```python
from build123d import *

# Parameters (mm, degrees)
SKETCH1_R                = 10
BOSS_EXTRUDE1_DEPTH      = 8
BOSS_EXTRUDE2_DEPTH      = 1.5
FILLET1_R                = 1.6
SKETCH5_R                = 10
SKETCH5_R_2              = 8
CUT_EXTRUDE1_DEPTH       = 5
CUT_EXTRUDE2_REACH       = 19.037
SKETCH6_R                = 1.2500000000000002
CIRPATTERN1_COUNT        = 4
CUT_EXTRUDE3_DEPTH       = 17.24807680927192
FILLET2_R                = 1.6
CIRPATTERN2_COUNT        = 2
FILLET2_OF_CIRPATTERN2_R = 1.6


with BuildPart() as part:
    # Sketch1 → Boss-Extrude1 (new body)
    with BuildSketch(Plane(origin=(0, 0, 0), x_dir=(1, 0, 0), z_dir=(0, 1, 0))):
        with Locations(Location((0, 0, 0), (0, 0, 270))):
            Circle(SKETCH1_R)
    extrude(amount=BOSS_EXTRUDE1_DEPTH)

    # Sketch4 → Boss-Extrude2 (add)
    with BuildSketch(Plane(origin=(0, 8, 0), x_dir=(1, 0, 0), z_dir=(0, 1, 0))):
        with BuildLine():
            Line((-1.449999999999999, 6.336205489092031), (-1.45, 1.9124591498905275))
            ThreePointArc((-1.45, 1.9124591498905275), (-2.4, 2.9e-16), (-1.45, -1.9124591498905275))
            Line((-1.45, -1.9124591498905275), (-1.449999999999999, -6.336205489092031))
            ThreePointArc((-1.449999999999999, -6.336205489092031), (4e-16, -6.499999999999999), (1.449999999999999, -6.336205489092031))
            Line((1.449999999999999, -6.336205489092031), (1.45, -1.9124591498905275))
            ThreePointArc((1.45, -1.9124591498905275), (2.4, 0), (1.45, 1.9124591498905275))
            Line((1.45, 1.9124591498905275), (1.449999999999999, 6.336205489092031))
            ThreePointArc((1.449999999999999, 6.336205489092031), (4e-16, 6.499999999999999), (-1.449999999999999, 6.336205489092031))
        make_face()
    extrude(amount=BOSS_EXTRUDE2_DEPTH)

    # Fillet1
    fillet1_edges = [part.edges().sort_by_distance(p)[0] for p in [
        (-1.4500000000000002, 8.75, -1.9124591498905277),
        (-1.4500000000000002, 8.75, 1.9124591498905277),
        (1.4500000000000002, 8.75, 1.9124591498905277),
        (1.4500000000000002, 8.75, -1.9124591498905277),
    ]]
    fillet(fillet1_edges, radius=FILLET1_R)

    # Sketch5 → Cut-Extrude1 (cut)
    with BuildSketch(Plane(origin=(0, 0, 0), x_dir=(1, 0, 0), z_dir=(0, 1, 0))):
        with Locations(Location((0, 0, 0), (0, 0, 270))):
            Circle(SKETCH5_R)
        with Locations(Location((0, 0, 0), (0, 0, 90))):
            Circle(SKETCH5_R_2, mode=Mode.SUBTRACT)
    extrude(amount=CUT_EXTRUDE1_DEPTH, mode=Mode.SUBTRACT)

    # Sketch6 → Cut-Extrude2 (cut, up to next)
    with BuildSketch(Plane.XZ, mode=Mode.PRIVATE) as cut_extrude2_sk1:
        with Locations(Location((4.242640687119277, 4.242640687119293, 0), (0, 0, 270))):
            Circle(SKETCH6_R)
    cut_extrude2_tool1 = extrude(cut_extrude2_sk1.sketch, amount=-CUT_EXTRUDE2_REACH, mode=Mode.PRIVATE) & part.part
    cut_extrude2 = cut_extrude2_tool1.solids().sort_by_distance((4.242641, 0, 4.242641))[0]
    add(cut_extrude2, mode=Mode.SUBTRACT)

    # CirPattern1: Cut-Extrude2 ×4 about axis
    cirpattern1_axis = Axis((7.37e-15, 0, -7.37e-15), (0, 1, 0))
    for i in range(1, CIRPATTERN1_COUNT):
        add(cut_extrude2.rotate(cirpattern1_axis, i * 360 / CIRPATTERN1_COUNT), mode=Mode.SUBTRACT)

    # Sketch7 → Cut-Extrude3 (cut, through all)
    with BuildSketch(Plane(origin=(0, 8, 0), x_dir=(1, 0, 0), z_dir=(0, 1, 0))):
        with BuildLine():
            Line((-3.233578363789502, -1.3393920132778183), (-7.852976026345933, -3.2528091751032733))
            ThreePointArc((-7.852976026345933, -3.2528091751032733), (-8.5, -1.04e-15), (-7.852976026345933, 3.2528091751032733))
            Line((-7.852976026345933, 3.2528091751032733), (-3.233578363789502, 1.3393920132778183))
            ThreePointArc((-3.233578363789502, 1.3393920132778183), (-3.5, -4.3e-16), (-3.233578363789502, -1.3393920132778183))
        make_face()
        with BuildLine():
            Line((-2.487442310373089, 6.005216961323361), (-3.826834323650907, 9.238795325112864))
            ThreePointArc((-3.826834323650907, 9.238795325112864), (6.1e-16, 10), (3.826834323650907, 9.238795325112864))
            Line((3.826834323650907, 9.238795325112864), (2.487442310373089, 6.005216961323361))
            ThreePointArc((2.487442310373089, 6.005216961323361), (4e-16, 6.5), (-2.487442310373089, 6.005216961323361))
        make_face()
    cut_extrude3 = extrude(amount=-CUT_EXTRUDE3_DEPTH, mode=Mode.SUBTRACT)

    # Fillet2
    fillet2_edges = [part.edges().sort_by_distance(p)[0] for p in [
        (-7.852976026345933, 6.5, 3.2528091751032733),
        (-7.852976026345933, 6.5, -3.2528091751032733),
        (-3.233578363789502, 4, 1.3393920132778185),
        (-3.233578363789502, 4, -1.3393920132778183),
        (2.487442310373089, 4, -6.005216961323361),
        (-2.4874423103730887, 4, -6.005216961323361),
        (3.826834323650907, 6.5, -9.238795325112866),
        (-3.826834323650907, 6.5, -9.238795325112866),
    ]]
    fillet(fillet2_edges, radius=FILLET2_R)

    # CirPattern2: Cut-Extrude3 ×2 about axis
    cirpattern2_axis = Axis((-8.01e-15, 0, 6.38e-15), (0, 1, 0))
    for i in range(1, CIRPATTERN2_COUNT):
        add(cut_extrude3.rotate(cirpattern2_axis, i * 360 / CIRPATTERN2_COUNT), mode=Mode.SUBTRACT)

    # Fillet2 of CirPattern2
    fillet2_of_cirpattern2_edges = [part.edges().sort_by_distance(p)[0] for p in [
        (7.852976026345917, 6.5, -3.2528091751032595),
        (7.852976026345917, 6.5, 3.252809175103287),
        (3.233578363789486, 4, -1.3393920132778052),
        (3.233578363789486, 4, 1.3393920132778316),
        (-2.487442310373106, 4, 6.005216961323374),
        (2.487442310373072, 4, 6.005216961323374),
        (-3.826834323650924, 6.5, 9.238795325112878),
        (3.8268343236508895, 6.5, 9.238795325112878),
    ]]
    fillet(fillet2_of_cirpattern2_edges, radius=FILLET2_OF_CIRPATTERN2_R)


solid = part.part
```
Can you work these out from the model? Positions are in its coordinate system, mm. A direction names the side the tool comes from. Give positions to 0.01 mm unless a question says otherwise; leave off trailing zeros. Loops run counter-clockwise (first coordinate to the right, second up) from the corner with the lowest first, then second, coordinate; pieces in that order, holes last. Notation, with made-up numbers: M 20,6.25 L 56,6.25 A13 ccw 56,17.25 Z; hole C -14,89.25 d2. An arc over 180 degrees is marked long. Answer in a Markdown table with one row per item.
1. Thinking about a two-plate mould opening in X: for faces 4 (the cylindrical face through (8.5, 6.5, 0)), 5 (the flat face through (0, 0, 0)), 6 (the cylindrical face through (5.9, 2.5, -5.4)), which applies, released by +X, released by -X, zero draft, split by the parting line, or undercut?
Taken from the geometry:
| item | result |
|---|---|
| face 4 | undercut |
| face 5 | zero draft |
| face 6 | released by +X |
2. Suppose I cut it at D-D on z = -7. Write out the boundary of the cut face in (x, y), plus the area to 3 significant figures.
Taken from the geometry:
| item | result |
|---|---|
| outline | M -7.14,5 L -3.87,5 L -3.87,0 L -2.85,0 L -2.85,8 L -7.14,8 Z; M 2.85,0 L 3.87,0 L 3.87,5 L 7.14,5 L 7.14,8 L 2.85,8 Z |
| area | 36.0 mm² |
3. Which directions (+Z, -Z, +X, -X, +Y, -Y) give clear straight access to the entire face, cutting with the end or side of a thin tool? Please do faces 1 (the cylindrical face through (-3.731, 3.944, -1.226)), 2 (the cylindrical face through (2.3, 4.68, 6.53)), 3 (the cylindrical face through (-2.4, 8.7, 0)).
Taken from the geometry:
| item | result |
|---|---|
| face 1 | +Y, -Y |
| face 2 | +Z, +Y, -Y |
| face 3 | -X, +Y |
4. For pin 1 Ø1.2 at (y, z) = (8.5, 4) entering from -X; pin 2 Ø1.5 at (x, z) = (4.24, -4.24) entering from -Y; pin 3 Ø1.5 at (y, z) = (8.5, 3) entering from +X; pin 4 Ø0.8 at (y, z) = (8.5, 3.5) entering from +X, each with a flat end and sliding along its axis, tell me the tip position at first contact or that it passes through.
Taken from the geometry:
| item | result |
|---|---|
| pin 1 | stops at x = -9.3 |
| pin 2 | passes through |
| pin 3 | stops at x = 9.7 |
| pin 4 | stops at x = 1.45 |
5. Suppose I cut it at C-C on x = 8. Write out the boundary of the cut face in (y, z).
Taken from the geometry:
| item | result |
|---|---|
| outline | M 5,-6 L 8,-6 L 8,-2.16 L 5,-2.16 Z; M 5,2.16 L 8,2.16 L 8,6 L 5,6 Z |
6. Suppose I cut it at B-B on y = 8.25. Write out the boundary of the cut face in (x, z).
Taken from the geometry:
| item | result |
|---|---|
| outline | M -1.83,-1.55 A1.6 cw -1.45,-2.59 L -1.45,-6.35 A1.6 cw -1.25,-6.38 A6.5 ccw 1.25,-6.38 A1.6 cw 1.45,-6.35 L 1.45,-2.59 A1.6 cw 1.83,-1.55 A2.4 ccw 1.83,1.55 A1.6 cw 1.45,2.59 L 1.45,6.35 A1.6 cw 1.25,6.38 A6.5 ccw -1.25,6.38 A1.6 cw -1.45,6.35 L -1.45,2.59 A1.6 cw -1.83,1.55 A2.4 ccw Z |
7. If I drill on line 1 along Z through (x, y) = (4.25, 2.25); line 2 along X through (y, z) = (6, -4.75); line 3 along X through (y, z) = (3.25, 5) (3 decimals), over which ranges is the centre line in solid material (lowest first)?
Taken from the geometry:
| item | result |
|---|---|
| line 1 | z = -6.78 to -5.49, -2.99 to -1.74, 1.74 to 2.99, 5.49 to 6.78 |
| line 2 | x = -8.8 to -5.39, -3.1 to 3.1, 5.39 to 8.8 |
| line 3 | x = -6.245 to -5.237, -3.248 to 3.248, 5.237 to 6.245 |
8. Suppose I cut it at A-A on z = 5. Write out the boundary of the cut face in (x, y) (3 decimals), plus the area to 3 significant figures.
Taken from the geometry:
| item | result |
|---|---|
| outline | M -8.66,5 L -6.245,5 L -6.245,0 L -5.237,0 L -5.237,8 L -8.66,8 Z; M -3.248,0 L 3.248,0 L 3.248,8 L 1.45,8 L 1.45,9.5 L -1.45,9.5 L -1.45,8 L -3.248,8 Z; M 5.237,0 L 6.245,0 L 6.245,5 L 8.66,5 L 8.66,8 L 5.237,8 Z |
| area | 86.9 mm² |
